Source: CAD feature listing. Evaluate the final solid. Frame: model axes, mm. A direction names the side the tool comes from. Give positions to 0.01 mm unless a question says otherwise; leave off trailing zeros. Loops run counter-clockwise (first coordinate to the right, second up) from the corner with the lowest first, then second, coordinate; pieces in that order, holes last. Notation, with made-up numbers: (55, 7) -> (64, 7) arc R22 ccw to (64, 34) -> close; hole circle Ø2 at (-18, 89). An arc over 180 degrees is marked (long way). Return JSON: item names as keys, results as strings. Group by question number.
(1) Ray query, line 1 (Y direction, x = 39.5, z = -12); line 2 (Z direction, x = -18.5, y = -3.5); line 3 (Z direction, x = -10, y = 7.5). Return the intervals inside material, ascending. Write a range as from..to.
(2) Pin query (flat end, axial travel): pin 1 (6 mm diameter, centred on y = 7, z = -14, fed in from -X); pin 2 (6 mm diameter, centred on x = 35, y = 2.5, fed in from -Z); pin 3 (1 mm diameter, centred on y = -2.5, z = -33.5, fed in from +X). Return the tip coordinate at first contact, or that it passes through.
(3) Draft query along Z for faces 3 (the face through (8.67, 3.45, 39.05)), 4 (the face through (-10, 5, 0)), 5 (the face through (-1, -7, 1)), 6 (the face through (15, 5, 20)). Return one class per face: released by +Z, released by -Z, zero draft, split by the parting line, or undercut.
(4) Access query for faces 1 (the face through (-30.2, 0, -26.5)), 2 (the face through (0, 10, 0)). Directions: +Z, -Z, +X, -X, +Y, -Y. A direction counts if a zero-diameter tool reaches every point of the face in a straight line with its end or side. Return the directions, or none.
(5) Cut plane B-B on z = 0. Return loops of the section in (x, y), then the cut area to 3 significant figures.
(6) Cut plane A-A on x = 0. Return loops of the section in (y, z), then the cut area to 3 significant figures.
(7) Cut plane D-D on y = -5. Return loops of the section in (x, z).
(8) Cut plane C-C on y = 1.75. Return loops of the section in (x, z).
Autodesk Inventor part; units mm, degrees
ref_plane "YZ Plane" through (0, 0, 0) normal (1, 0, 0) x (0, 1, 0)
ref_plane "XZ Plane" through (0, 0, 0) normal (0, 1, 0) x (-1, 0, 0)
ref_plane "XY Plane" through (0, 0, 0) normal (0, 0, 1) x (1, 0, 0)
sketch "Sketch1" plane through (0, 0, 0) normal (0, 1, 0) x (-1, 0, 0)
  circle A0 centre (0, 0) radius 40
  circle A1 centre (0, 0) radius 35
  dimension "d0" = 80
  dimension "d1" = 70
extrude "Extrusion1" add sketch "Sketch1" along normal blind 10 contours A1
extrude "Extrusion2" add sketch "Sketch1" along normal blind 7
sketch "Sketch3" plane through (0, 0, 0) normal (0, -1, 0) x (1, 0, 0)
  circle A0 centre (0, 0) radius 45
  dimension "d14" = 90
extrude "Extrusion4" add sketch "Sketch3" along normal blind 7
fillet "Fillet1" radius 4 1 edges at (-45, -7, 0)
sketch "Sketch4" plane through (0, 10, 0) normal (0, 1, 0) x (1, 0, 0)
  circle A0 centre (14.9762, -20.0178) radius 12
  circle A1 centre (-10, 0) radius 27
  circle A2 centre (14.9762, -20.0178) radius 1.25
  circle A3 centre (-10, 0) radius 1.25
  point P0 (0, 0)
  dimension "d24" = 24
  dimension "d25" = 54
  dimension "d26" = 10
  dimension "d27" = 2.5
  dimension "d28" = 2.5
  dimension "d31" = 25
extrude "Extrusion5" cut sketch "Sketch4" against normal blind 5 contours A2 | A3
properties part number "Cap"
Answers:
{
 "1": {"line 1": "-6.99..0", "line 2": "-40.99..40.99", "line 3": "-33.54..-1.25, 1.25..33.54"},
 "2": {"pin 1": "x = -38.46", "pin 2": "z = -30.22", "pin 3": "x = 30.59"},
 "3": {"face 3": "split by the parting line", "face 4": "undercut", "face 5": "zero draft", "face 6": "undercut"},
 "4": {"face 1": "+Y", "face 2": "+Z, -Z, +X, -X, +Y"},
 "5": {"outline": "(-45, -3) arc R4 ccw to (-41, -7) -> (41, -7) arc R4 ccw to (45, -3) -> (45, 0) -> (40, 0) -> (40, 7) -> (35, 7) -> (35, 10) -> (-8.75, 10) -> (-8.75, 5) -> (-11.25, 5) -> (-11.25, 10) -> (-35, 10) -> (-35, 7) -> (-40, 7) -> (-40, 0) -> (-45, 0) -> close", "area": "1,380 mm²"},
 "6": {"outline": "(-7, -41) arc R4 ccw to (-3, -45) -> (0, -45) -> (0, -40) -> (7, -40) -> (7, -35) -> (10, -35) -> (10, 35) -> (7, 35) -> (7, 40) -> (0, 40) -> (0, 45) -> (-3, 45) arc R4 ccw to (-7, 41) -> close", "area": "1,390 mm²"},
 "7": {"outline": "circle Ø88.93 at (0, 0)"},
 "8": {"outline": "circle Ø80 at (0, 0)"}
}
